```python
from build123d import *

# Parameters (mm, degrees)
BOSS_EXTRUDE1_DEPTH = 6.35
SKETCH3_W           = 12.7
SKETCH3_H           = 36.83
CUT_EXTRUDE1_DEPTH  = 6.35


with BuildPart() as part:
    # Sketch1 → Boss-Extrude1 (new body)
    with BuildSketch(Plane.XY):
        Polygon((10.16, 0.022003094), (10.16, 44.472003094), (1.27, 44.472003094), (1.27, 54.632003094), (-1.27, 54.632003094), (-1.27, 44.472003094), (-10.16, 44.472003094), (-10.16, 0.022003094), (-1.27, 0.022003094), (-1.27, -6.327996906), (1.27, -6.327996906), (1.27, 0.022003094), align=None)
    extrude(amount=BOSS_EXTRUDE1_DEPTH)

    # Sketch3 → Cut-Extrude1 (cut)
    with BuildSketch(Plane.XY.offset(6.35)):
        with Locations((0, 22.247003094)):
            Rectangle(SKETCH3_W, SKETCH3_H)
    extrude(amount=-CUT_EXTRUDE1_DEPTH, mode=Mode.SUBTRACT)


solid = part.part
```
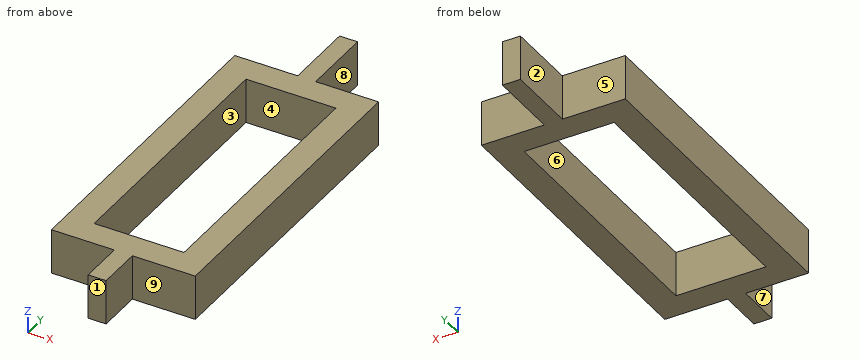
Can you work these out from the model? Positions are in its coordinate system, mm. Face numbers are marked on the shaded views. A direction names the side the tool comes from. Give positions to 0.01 mm unless a question says otherwise; leave off trailing zeros. Loops run counter-clockwise (first coordinate to the right, second up) from the corner with the lowest first, then second, coordinate; pieces in that order, holes last. Notation, with made-up numbers: M -19,-10.5 L 26,-10.5 A25 cw 26,9.5 Z; hole C 81,11 d6. An arc over 180 degrees is marked long. Use one line per item in the form item = value. Start each with the question number.
(1) I'm going to push flat-ended pins straight in: P1, Ø1.9, axis at y = -2, z = 2, coming from the +X side; P2, Ø1.5, axis at x = -5, z = 1, coming from the -Y side; P3, Ø2, axis at x = 6, z = 4, coming from the +Y side. Where does each tip first touch, or does it pass through?
(2) On a 3-axis mill with a long thin cutter (end or side, diameter ignored), from which of +Z, -Z, +X, -X, +Y, -Y can I reach the whole of each face in a straight line? I mean the marked faces 5, 6, 7, 8 and 9. Say none if no direction works.
(3) Please list where these lines run through material, in increasing order: line 1 (Y direction, x = 5, z = 2.75); line 2 (X direction, y = 12.5, z = 1.5); line 3 (Y direction, x = -0.25, z = 3.25).
(4) Thinking about a two-plate mould opening in Y: for the marked faces 1, 2, 3 and 4, which applies, released by +Y, released by -Y, zero draft, split by the parting line, or undercut?
(5) I want a section at D-D, the plane x = -7.5. Write out the boundary of the cut face in (y, z).
(6) I want a section at B-B, the plane x = -2. Write out the boundary of the cut face in (y, z).
(7) I want a section at A-A, the plane y = 12.5. Write out the boundary of the cut face in (x, z), and give its area (3 significant figures).
(8) I want a section at C-C, the plane z = 3. Write out the boundary of the cut face in (x, y), and give its area (3 significant figures).
Worked out:
q1.P1 = 1.27
q1.P2 = 0.02
q1.P3 = 44.47
q2.face_5 = +Z, -Z, -X, +Y
q2.face_6 = +Z, -Z
q2.face_7 = +Z, -Z, -X, -Y
q2.face_8 = +Z, -Z, +X, +Y
q2.face_9 = +Z, -Z, +X, -Y
q3.line_1 = 0.02 to 3.83, 40.66 to 44.47
q3.line_2 = -10.16 to -6.35, 6.35 to 10.16
q3.line_3 = -6.33 to 3.83, 40.66 to 54.63
q4.face_1 = released by -Y
q4.face_2 = zero draft
q4.face_3 = undercut
q4.face_4 = undercut
q5.outline = M 0.02,0 L 44.47,0 L 44.47,6.35 L 0.02,6.35 Z
q6.outline = M 0.02,0 L 3.83,0 L 3.83,6.35 L 0.02,6.35 Z; M 40.66,0 L 44.47,0 L 44.47,6.35 L 40.66,6.35 Z
q7.outline = M -10.16,0 L -6.35,0 L -6.35,6.35 L -10.16,6.35 Z; M 6.35,0 L 10.16,0 L 10.16,6.35 L 6.35,6.35 Z
q7.area = 48.4 mm²
q8.outline = M -10.16,0.02 L -1.27,0.02 L -1.27,-6.33 L 1.27,-6.33 L 1.27,0.02 L 10.16,0.02 L 10.16,44.47 L 1.27,44.47 L 1.27,54.63 L -1.27,54.63 L -1.27,44.47 L -10.16,44.47 Z; hole M -6.35,3.83 L 6.35,3.83 L 6.35,40.66 L -6.35,40.66 Z
q8.area = 477 mm²
